Can you work these out from the model? Positions are in its coordinate system, mm. Face numbers are marked on the shaded views. A direction names the side the tool comes from. Round coordinates to 2 decimals unless told otherwise and drop trailing zeros. Write each loop counter-clockwise with the first axis right and the second up, starting at its lowest first coordinate (ties: lowest second). Pieces come first, ordered by that corner, then holes. Notation, with made-up numbers: M 52,19 L 101,19 A25 ccw 101,39 Z; hole C -23,-6.75 d1. An arc over 180 degrees is marked long. Answer as a JSON object with one key per item and string values. Group by question number.
1) Suppose I cut it at A-A, the plane x = -7.7. Write out the boundary of the cut face in (y, z).
2) I'm going to push flat-ended pins straight in: pin 1 Ø2 at (y, z) = (-26, 19.5) entering from +X; pin 2 Ø1.5 at (y, z) = (-16.5, 17.5) entering from -X; pin 3 Ø1.6 at (x, z) = (-10.5, 0.5) entering from -Y. Where does each tip first touch, or does it pass through?
3) Please list where these lines run through material, in increasing order: L1, parallel to X at y = -40, z = 1; L2, parallel to Y at x = 156.3, z = 1.45; L3, parallel to X at y = -44.5, z = 10.5. Write a range as [from, to].
4) Suppose I cut it at D-D, the plane x = 150.5. Write out the boundary of the cut face in (y, z).
5) On a 3-axis mill with a long thin cutter (end or side, diameter ignored), from which of +Z, -Z, +X, -X, +Y, -Y can I reach the whole of each face in a straight line? I mean the marked faces 1 and 2. Say none if no direction works.
6) Suppose I cut it at B-B, the plane y = -40.9. Write out the boundary of the cut face in (x, z).
7) Suppose I cut it at C-C, the plane y = -14.5. Write out the boundary of the cut face in (x, z).
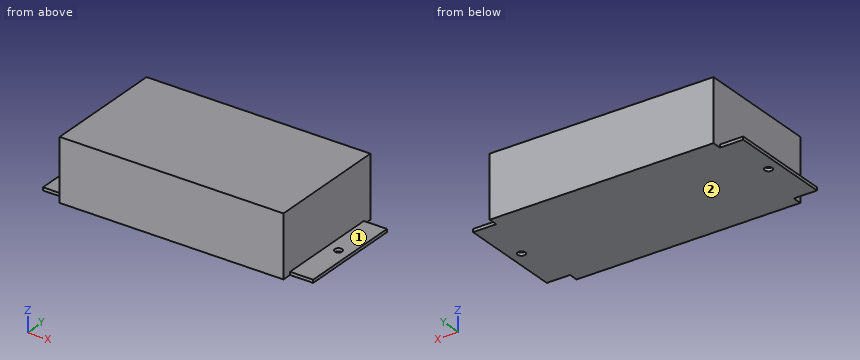
from build123d import *

# Parameters (mm, degrees)
SKETCH1_W           = 148.6
SKETCH1_H           = 81.8
BOSS_EXTRUDE1_DEPTH = 41
SKETCH2_W           = 15.4
SKETCH2_H           = 69.5
SKETCH2_R           = 2.5
BOSS_EXTRUDE2_DEPTH = 2


with BuildPart() as part:
    # Sketch1 → Boss-Extrude1 (new body)
    with BuildSketch(Plane.XY):
        with Locations((74.3, -40.9)):
            Rectangle(SKETCH1_W, SKETCH1_H)
    extrude(amount=BOSS_EXTRUDE1_DEPTH)

    # Sketch2 → Boss-Extrude2 (add)
    with BuildSketch(Plane(origin=(0, 0, 0), x_dir=(-1, 0, 0), z_dir=(0, 0, -1))):
        with Locations((7.7, -40.9)):
            Rectangle(SKETCH2_W, SKETCH2_H)
        with Locations((7.7, -40.9)):
            Circle(SKETCH2_R, mode=Mode.SUBTRACT)
        with Locations((-156.3, -40.9)):
            Rectangle(SKETCH2_W, SKETCH2_H)
        with Locations((-156.3, -40.9)):
            Circle(SKETCH2_R, mode=Mode.SUBTRACT)
    extrude(amount=-BOSS_EXTRUDE2_DEPTH)


solid = part.part
Results:
{
 "1": {"outline": "M -75.65,0 L -43.4,0 L -43.4,2 L -75.65,2 Z; M -38.4,0 L -6.15,0 L -6.15,2 L -38.4,2 Z"},
 "2": {"pin 1": "x = 148.6", "pin 2": "x = 0", "pin 3": "y = -75.65"},
 "3": {"L1": "[-15.4, -10.03], [-5.37, 153.97], [158.63, 164]", "L2": "[-75.65, -43.4], [-38.4, -6.15]", "L3": "[0, 148.6]"},
 "4": {"outline": "M -75.65,0 L -6.15,0 L -6.15,2 L -75.65,2 Z"},
 "5": {"face 1": "+Z, +X, +Y, -Y", "face 2": "-Z, +X, -X, +Y, -Y"},
 "6": {"outline": "M -15.4,0 L -10.2,0 L -10.2,2 L -15.4,2 Z; M -5.2,0 L 153.8,0 L 153.8,2 L 148.6,2 L 148.6,41 L 0,41 L 0,2 L -5.2,2 Z; M 158.8,0 L 164,0 L 164,2 L 158.8,2 Z"},
 "7": {"outline": "M -15.4,0 L 164,0 L 164,2 L 148.6,2 L 148.6,41 L 0,41 L 0,2 L -15.4,2 Z"}
}
